For this review, take the finished solid that the model builds, in its own axes (mm). Face numbers are marked on the shaded views. A direction names the side the tool comes from. Give positions to 0.01 mm unless a question says otherwise; leave off trailing zeros. Loops run counter-clockwise (first coordinate to the right, second up) from the corner with the lowest first, then second, coordinate; pieces in that order, holes last. Notation, with made-up numbers: (49.5, 45.25) -> (88.5, 45.25) arc R31 ccw to (88.5, 81.25) -> close; hole circle Ø3 at (61, 76). An arc over 180 degrees is marked (long way). One line per question, with ' | ' between items. Start each with the question number.
(1) Consider section D-D (x = -0.95). Write out the cut boundary in (y, z), and give its area (3 significant figures).
(2) Insertion check: P1, Ø1.5, axis at y = 1, z = -0.5, coming from the +X side; P2, Ø1.6, axis at x = -0.5, y = 5.5, coming from the +Z side; P3, Ø1.5, axis at x = 1, z = 0.5, coming from the +Y side. Each pin has a flat end and moves straight along its axis. Give the tip position at first contact, or say it passes through.
(3) Consider section C-C (z = 1.35). Write out the cut boundary in (x, y), and give its area (3 significant figures).
(4) Tool access review of the marked faces 1, 2, 3 and 4: name each direction out of +Z, -Z, +X, -X, +Y, -Y from which nothing blocks a thin tool from reaching the whole face with its end or side.
(5) Wall thickness on probe 1 along Z at (x, y) = (-0.95, 2); probe 2 along X at (y, z) = (7.75, 0.05); probe 3 along Z at (x, y) = (-1.1, 6.75): over which ranges is each line inside the solid? List them lowest first.
(6) Consider section A-A (x = -0.3). Write out the cut boundary in (y, z).
(7) Consider section B-B (y = 0.25). Write out the cut boundary in (x, z).
(8) Draft analysis for pull direction Y (two halves, no side actions). For the marked faces 5, 6, 7 and 8, state which applies: +Y half, -Y half, draft (parallel to the pull), parting line (faces both ways), or undercut.
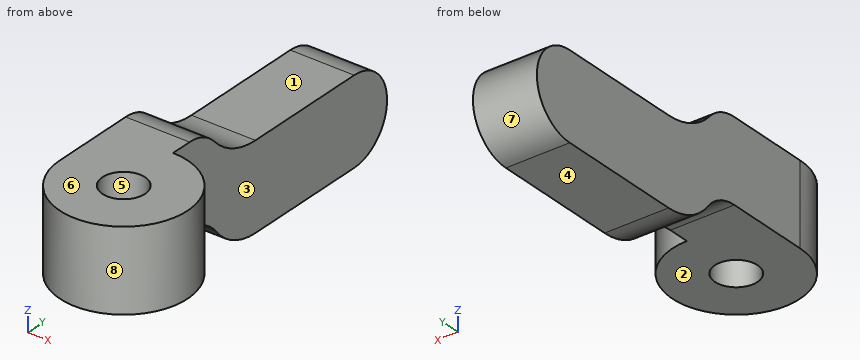
from build123d import *

# Parameters (mm, degrees)
CROQUIS1_R              = 1.5
CROQUIS1_R_2            = 0.5
SALIENTE_EXTRUIR1_DEPTH = 1.9
SALIENTE_EXTRUIR2_DEPTH = 1.5
SALIENTE_EXTRUIR3_START = -1.9
SALIENTE_EXTRUIR3_DEPTH = 1.9


with BuildPart() as part:
    # Croquis1 → Saliente-Extruir1 (new body)
    with BuildSketch(Plane.XY):
        with Locations(Location((0, 0, 0), (0, 0, 180))):
            Circle(CROQUIS1_R)
        Circle(CROQUIS1_R_2, mode=Mode.SUBTRACT)
    extrude(amount=SALIENTE_EXTRUIR1_DEPTH)

    # Croquis2 → Saliente-Extruir2 (add)
    with BuildSketch(Plane(origin=(0, 0, 0), x_dir=(0, 0, -1), z_dir=(1, 0, 0))):
        with BuildLine():
            Line((-1.9, 2), (-1.9, 1))
            Line((-1.9, 1), (0, 1))
            Line((0, 1), (0, 2))
            ThreePointArc((0, 2), (0.105572809, 2.447213595), (0.4, 2.8))
            ThreePointArc((0.4, 2.8), (0.841640786, 3.329179607), (1, 4))
            Line((1, 4), (1, 7))
            ThreePointArc((1, 7), (0, 8), (-1, 7))
            Line((-1, 7), (-1, 4))
            ThreePointArc((-1, 4), (-1.147286816, 3.313779067), (-1.563201663, 2.748440748))
            ThreePointArc((-1.563201663, 2.748440748), (-1.811921505, 2.410364677), (-1.9, 2))
        make_face()
    extrude(amount=-SALIENTE_EXTRUIR2_DEPTH)

    # Croquis3 → Saliente-Extruir3 (add)
    with BuildSketch(Plane.XY.offset(1.9).offset(SALIENTE_EXTRUIR3_START)):
        with BuildLine():
            Line((-1.5, 1), (-1.5, 0))
            ThreePointArc((-1.5, 0), (-1.401258538, 0.535233135), (-1.118033989, 1))
            Line((-1.118033989, 1), (-1.5, 1))
        make_face()
    extrude(amount=SALIENTE_EXTRUIR3_DEPTH)


solid = part.part
A:
1) outline: (-1.16, 0) -> (2, 0) arc R1 cw to (2.8, -0.4) arc R1.5 ccw to (4, -1) -> (7, -1) arc R1 ccw to (7, 1) -> (4, 1) arc R1.67 cw to (2.75, 1.56) arc R1 ccw to (2, 1.9) -> (-1.16, 1.9) -> close | area: 17.5 mm^2
2) P1: stops at x = 1.43 | P2: stops at z = 1 | P3: stops at y = 1.48
3) outline: (-1.5, 0) arc R1.5 ccw (long way) to (0, 1.5) -> (0, 2.98) -> (-1.5, 2.98) -> close; hole circle Ø1 at (0, 0) | area: 8.98 mm^2
4) face 1: +Z, +X, -X, +Y | face 2: -Z, +X, -X, -Y | face 3: +Z, -Z, +X, +Y | face 4: -Z, +X, -X, +Y, -Y
5) probe 1: z = 0 to 1.9 | probe 2: x = -1.5 to 0 | probe 3: z = -1 to 1
6) outline: (-1.47, 0) -> (-0.4, 0) -> (-0.4, 1.9) -> (-1.47, 1.9) -> close; (0.4, 0) -> (2, 0) arc R1 cw to (2.8, -0.4) arc R1.5 ccw to (4, -1) -> (7, -1) arc R1 ccw to (7, 1) -> (4, 1) arc R1.67 cw to (2.75, 1.56) arc R1 ccw to (2, 1.9) -> (0.4, 1.9) -> close
7) outline: (-1.5, 0) -> (-0.43, 0) -> (-0.43, 1.9) -> (-1.5, 1.9) -> close; (0.43, 0) -> (1.48, 0) -> (1.48, 1.9) -> (0.43, 1.9) -> close
8) face 5: undercut | face 6: draft | face 7: +Y half | face 8: parting line
